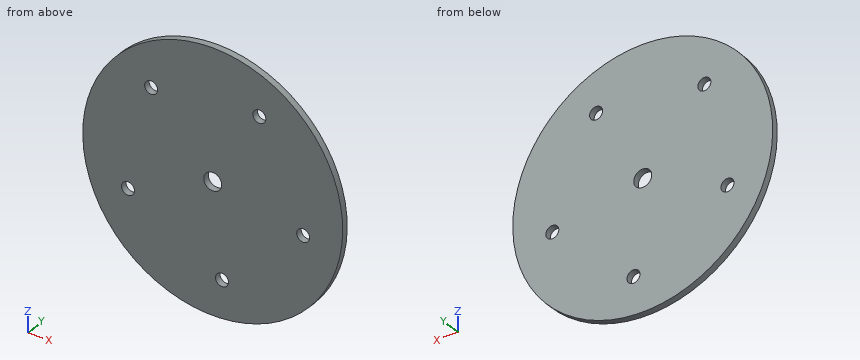
```python
from build123d import *

# Parameters (mm, degrees)
SKETCH1_R           = 60
BOSS_EXTRUDE1_DEPTH = 3
SKETCH2_R           = 4.15
CUT_EXTRUDE1_DEPTH  = 5
SKETCH3_R           = 3
CUT_EXTRUDE2_DEPTH  = 10


with BuildPart() as part:
    # Sketch1 → Boss-Extrude1 (new body)
    with BuildSketch(Plane(origin=(0, 0, 0), x_dir=(1, 0, 0), z_dir=(0, 1, 0))):
        with Locations(Location((0, 0, 0), (0, 0, 270))):
            Circle(SKETCH1_R)
    extrude(amount=BOSS_EXTRUDE1_DEPTH)

    # Sketch2 → Cut-Extrude1 (cut)
    with BuildSketch(Plane(origin=(0, 3, 0), x_dir=(1, 0, 0), z_dir=(0, 1, 0))):
        with Locations(Location((0, 0, 0), (0, 0, 270))):
            Circle(SKETCH2_R)
    extrude(amount=-CUT_EXTRUDE1_DEPTH, mode=Mode.SUBTRACT)

    # Sketch3 → Cut-Extrude2 (cut)
    with BuildSketch(Plane(origin=(0, 3, 0), x_dir=(1, 0, 0), z_dir=(0, 1, 0))):
        with Locations(Location((-28.451614764, -31.883278826, 0), (0, 0, 270))):
            Circle(SKETCH3_R)
        with Locations(Location((-39.114832567, 17.206618627, 0), (0, 0, 270))):
            Circle(SKETCH3_R)
        with Locations(Location((4.277318773, 42.517553969, 0), (0, 0, 270))):
            Circle(SKETCH3_R)
        with Locations(Location((41.75836095, 9.070674844, 0), (0, 0, 270))):
            Circle(SKETCH3_R)
        with Locations(Location((21.530767608, -36.911568614, 0), (0, 0, 270))):
            Circle(SKETCH3_R)
    extrude(amount=-CUT_EXTRUDE2_DEPTH, mode=Mode.SUBTRACT)


solid = part.part
```
The model under review builds one solid part; all positions refer to its coordinate system, in mm. Coordinates: 2 decimals unless noted, no trailing zeros. Write each loop counter-clockwise with the first axis right and the second up, starting at its lowest first coordinate (ties: lowest second). Pieces come first, ordered by that corner, then holes. Notation, with made-up numbers: (76, 44.5) - (127, 44.5) arc R17 ccw to (127, 55.5) - close; hole circle Ø7 at (-18.5, 21.5). An arc over 180 degrees is marked (long way). Answer in a Markdown table with one row per item. Add a question column.
Q1. To check wall thickness, follow line 1 along X through (y, z) = (2.45, 0); line 2 along X through (y, z) = (2.9, -11); line 3 along X through (y, z) = (0.8, -14). State the ranges of each line that lie inside material, in increasing order. Write a range as from..to.
Q2. Clearance check with flat-ended pins moving along their axes: pin 1 (1 mm diameter, centred on y = 1, z = -46, fed in from -X); pin 2 (1.5 mm diameter, centred on y = 2.5, z = -9.5, fed in from -X); pin 3 (1.5 mm diameter, centred on y = 1.5, z = 3, fed in from -X). State where each tip first meets the part, or that it passes through.
Q3. Consider section A-A on z = 0. Give the boundary of the cut face in (x, y).
Q4. Consider section B-B on y = 1.45. Give the boundary of the cut face in (x, z), then the cut area to 3 significant figures.
Q5. Consider section C-C on x = 17. Give the boundary of the cut face in (y, z), then the cut area to 3 significant figures.
Q6. Consider section D-D on z = -51.5. Give the boundary of the cut face in (x, y), then the cut area to 3 significant figures.
Answers below:
| question | item | result |
|---|---|---|
| 1 | line 1 | -60..-4.15, 4.15..60 |
| 1 | line 2 | -58.98..39.46, 44.06..58.98 |
| 1 | line 3 | -58.34..58.34 |
| 2 | pin 1 | x = -39.11 |
| 2 | pin 2 | x = -59.36 |
| 2 | pin 3 | x = -59.96 |
| 3 | outline | (-60, 0) - (-4.15, 0) - (-4.15, 3) - (-60, 3) - close; (4.15, 0) - (60, 0) - (60, 3) - (4.15, 3) - close |
| 4 | outline | circle Ø120 at (0, 0); hole circle Ø6 at (-39.11, -17.21); hole circle Ø6 at (-28.45, 31.88); hole circle Ø8.3 at (0, 0); hole circle Ø6 at (4.28, -42.52); hole circle Ø6 at (21.53, 36.91); hole circle Ø6 at (41.76, -9.07) |
| 4 | area | 11,100 mm² |
| 5 | outline | (0, -57.54) - (3, -57.54) - (3, 57.54) - (0, 57.54) - close |
| 5 | area | 345 mm² |
| 6 | outline | (-30.79, 0) - (30.79, 0) - (30.79, 3) - (-30.79, 3) - close |
| 6 | area | 185 mm² |
